Design review of the part built by this model. Coordinates are the model's own, in mm. Face numbers are marked on the shaded views. A direction names the side the tool comes from. Round coordinates to 2 decimals unless told otherwise and drop trailing zeros. Loops run counter-clockwise (first coordinate to the right, second up) from the corner with the lowest first, then second, coordinate; pieces in that order, holes last. Notation, with made-up numbers: (43, 54) - (68, 54) arc R28 cw to (68, 77) - close; hole circle Ø3 at (14.25, 23.5). An arc over 180 degrees is marked (long way). Use one line per item in the form item = value. Start each with the question number.
(1) Wall thickness on probe 1 along X at (y, z) = (1, 5.5); probe 2 along X at (y, z) = (3.5, -5.5); probe 3 along Z at (x, y) = (-32.5, 4.5): over which ranges is each line inside the solid? List them lowest first. Write a range as [from, to].
(2) Machinability: for the marked faces 1, 2 and 3, which of the approach directions +Z, -Z, +X, -X, +Y, -Y give a long, thin tool a straight path to every point of the face, cutting with its end or side? Answer none if there is none.
(3) We need section A-A, the plane y = 3.75. Write out the cut boundary in (x, z).
(4) The part is to be moulded in two halves that separate along Z. For the marked faces 4, 5, 6 and 7, say which applies: released by +Z, released by -Z, zero draft, split by the parting line, or undercut.
(5) We need section B-B, the plane z = -5.5. Write out the cut boundary in (x, y), then the cut area to 3 significant figures.
(6) We need section D-D, the plane x = -20. Write out the cut boundary in (y, z), then the cut area to 4 significant figures.
(7) For pin 1 (5 mm diameter, centred on x = -20.5, z = 4.5, fed in from +Y); pin 2 (0.8 mm diameter, centred on x = -24.5, y = 3.5, fed in from -Z); pin 3 (6 mm diameter, centred on x = -9.5, z = -3.5, fed in from +Y); pin 4 (1.4 mm diameter, centred on y = 7.5, z = -10, fed in from +X), all flat-tipped, find the tip position at first contact; note any pin that passes through.
(8) We need section C-C, the plane y = 8.25. Write out the cut boundary in (x, z), then the cut area to 3 significant figures.
from build123d import *

# Parameters (mm, degrees)
SKETCH5_W           = 40
SKETCH5_H           = 13
BOSS_EXTRUDE2_DEPTH = 10.5
SKETCH6_R           = 6.5
CUT_EXTRUDE4_DEPTH  = 8.5
SKETCH7_R           = 2.5
CUT_EXTRUDE5_DEPTH  = 4.5
SKETCH8_R           = 4
CUT_EXTRUDE6_DEPTH  = 5
CHAMFER8_SIZE       = 11
SKETCH9_W           = 2.5
SKETCH9_H           = 1.8
CUT_EXTRUDE7_DEPTH  = 15


with BuildPart() as part:
    # Sketch5 → Boss-Extrude2 (new body)
    with BuildSketch(Plane.XY):
        with Locations((-20, 6.5)):
            Rectangle(SKETCH5_W, SKETCH5_H)
    boss_extrude2 = extrude(amount=BOSS_EXTRUDE2_DEPTH)

    # Sketch6 → Cut-Extrude4 (cut)
    with BuildSketch(Plane(origin=(0, 0, 0), x_dir=(-1, 0, 0), z_dir=(0, 0, -1))):
        with Locations((20, 13)):
            Circle(SKETCH6_R)
    cut_extrude4 = extrude(amount=-CUT_EXTRUDE4_DEPTH, mode=Mode.SUBTRACT)

    # Sketch7 → Cut-Extrude5 (cut)
    with BuildSketch(Plane.XY.offset(10.5)):
        with Locations((-20, 13)):
            Circle(SKETCH7_R)
    cut_extrude5 = extrude(amount=-CUT_EXTRUDE5_DEPTH, mode=Mode.SUBTRACT)

    # Mirror5: Boss-Extrude2, Cut-Extrude4, Cut-Extrude5 across plane
    add(boss_extrude2.mirror(Plane.XY))
    add(cut_extrude4.mirror(Plane.XY), mode=Mode.SUBTRACT)
    add(cut_extrude5.mirror(Plane.XY), mode=Mode.SUBTRACT)

    # Sketch8 → Cut-Extrude6 (cut)
    with BuildSketch(Plane.XZ):
        with Locations(Location((-31, 5.5, 0), (0, 0, 270))):
            Circle(SKETCH8_R)
        with Locations(Location((-9, 5.5, 0), (0, 0, 90))):
            Circle(SKETCH8_R)
        with Locations(Location((-9, -5.5, 0), (0, 0, 270))):
            Circle(SKETCH8_R)
        with Locations(Location((-31, -5.5, 0), (0, 0, 90))):
            Circle(SKETCH8_R)
    extrude(amount=-CUT_EXTRUDE6_DEPTH, mode=Mode.SUBTRACT)

    # Chamfer8
    chamfer8_edges = [part.edges().sort_by_distance(p)[0] for p in [
        (-40, 13, 0),
        (0, 13, 0),
    ]]
    chamfer(chamfer8_edges, length=CHAMFER8_SIZE)

    # Sketch9 → Cut-Extrude7 (cut)
    with BuildSketch(Plane.XZ):
        with Locations((-15.75, 9.6)):
            Rectangle(SKETCH9_W, SKETCH9_H)
        with Locations((-24.25, 9.6)):
            Rectangle(SKETCH9_W, SKETCH9_H)
        with Locations((-15.75, -9.6)):
            Rectangle(SKETCH9_W, SKETCH9_H)
        with Locations((-24.25, -9.6)):
            Rectangle(SKETCH9_W, SKETCH9_H)
    extrude(amount=-CUT_EXTRUDE7_DEPTH, mode=Mode.SUBTRACT)


solid = part.part
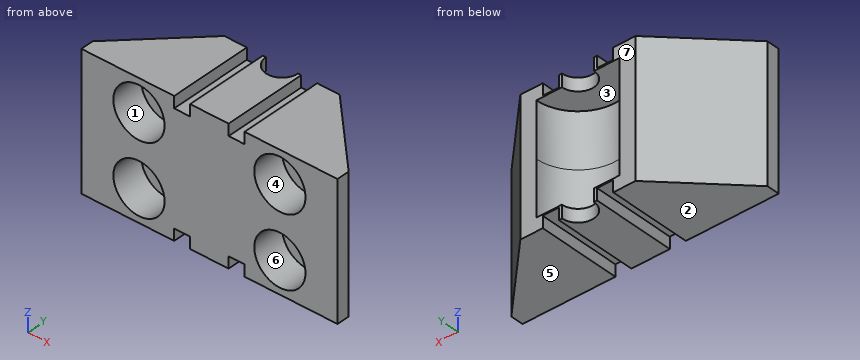
Data:
q1.probe_1 = [-40, -35], [-27, -13], [-5, 0]
q1.probe_2 = [-38.5, -35], [-27, -13], [-5, -1.5]
q1.probe_3 = [-10.5, -9.21], [-1.79, 1.79], [9.21, 10.5]
q2.face_1 = -Y
q2.face_2 = -Z, +X, -X, +Y, -Y
q2.face_3 = +Y
q3.outline = (-38.25, -10.5) - (-25.5, -10.5) - (-25.5, -8.7) - (-23, -8.7) - (-23, -10.5) - (-17, -10.5) - (-17, -8.7) - (-14.5, -8.7) - (-14.5, -10.5) - (-1.75, -10.5) - (-1.75, 10.5) - (-14.5, 10.5) - (-14.5, 8.7) - (-17, 8.7) - (-17, 10.5) - (-23, 10.5) - (-23, 8.7) - (-25.5, 8.7) - (-25.5, 10.5) - (-38.25, 10.5) - close; hole circle Ø8 at (-31, -5.5); hole circle Ø8 at (-31, 5.5); hole circle Ø8 at (-9, -5.5); hole circle Ø8 at (-9, 5.5)
q4.face_4 = undercut
q4.face_5 = released by -Z
q4.face_6 = undercut
q4.face_7 = zero draft
q5.outline = (-40, 0) - (-35, 0) - (-35, 5) - (-27, 5) - (-27, 0) - (-13, 0) - (-13, 5) - (-5, 5) - (-5, 0) - (0, 0) - (0, 2) - (-11, 13) - (-13.5, 13) arc R6.5 cw to (-26.5, 13) - (-29, 13) - (-40, 2) - close
q5.area = 253 mm^2
q6.outline = (0, -10.5) - (10.5, -10.5) - (10.5, -8.5) - (6.5, -8.5) - (6.5, 8.5) - (10.5, 8.5) - (10.5, 10.5) - (0, 10.5) - close
q6.area = 152.5 mm^2
q7.pin_1 = 7.23
q7.pin_2 = -8.7
q7.pin_3 = 13
q7.pin_4 = -4.8
q8.outline = (-33.75, -10.5) - (-25.5, -10.5) - (-25.5, -8.7) - (-23, -8.7) - (-23, -10.5) - (-17, -10.5) - (-17, -8.7) - (-14.5, -8.7) - (-14.5, -10.5) - (-6.25, -10.5) - (-6.25, 10.5) - (-14.5, 10.5) - (-14.5, 8.7) - (-17, 8.7) - (-17, 10.5) - (-23, 10.5) - (-23, 8.7) - (-25.5, 8.7) - (-25.5, 10.5) - (-33.75, 10.5) - close; hole (-24.44, -8.5) - (-15.56, -8.5) - (-15.56, 8.5) - (-24.44, 8.5) - close
q8.area = 409 mm^2
